```python
from build123d import *

# Parameters (mm, degrees)
F1_DEPTH = 50
F3_DEPTH = 3
F5_DEPTH = 3


with BuildPart() as f1:
    # F0 (on Front) → F1 (new body)
    with BuildSketch(Plane.XZ):
        Polygon((300, 0), (0, 0), (0, -3), (298.757359, -3), (474.655375, -178.898016), (476.776695, -176.776695), align=None)
    extrude(amount=F1_DEPTH)

    # F2 (on face) → F3 (join)
    with BuildSketch(Plane.XZ.offset(50)):
        Polygon((474.655375, -178.898016), (298.757359, -3), (0, -3), (0, -50), (279.289322, -50), (441.421356, -212.132034), align=None)
    extrude(amount=-F3_DEPTH)

    # F4 (on face) → F5 (join)
    with BuildSketch(Plane(origin=(0, 0, 0), x_dir=(-1, 0, 0), z_dir=(0, 1, 0))):
        Polygon((-298.757359, -3), (-474.655375, -178.898016), (-441.421356, -212.132034), (-279.289322, -50), (0, -50), (0, -3), align=None)
    extrude(amount=-F5_DEPTH)


solid = f1.part
```
Can you work these out from the model? Positions are in its coordinate system, mm. A direction names the side the tool comes from. Give positions to 0.01 mm unless a question says otherwise; leave off trailing zeros. Loops run counter-clockwise (first coordinate to the right, second up) from the corner with the lowest first, then second, coordinate; pieces in that order, holes last. Notation, with made-up numbers: M -4.5,67.5 L 53.5,67.5 A35 cw 53.5,101.5 Z; hole C 56.25,-10.5 d2. An arc over 180 degrees is marked long. Use one line per item in the form item = value. Start each with the question number.
(1) Please list where these lines run through material, in increasing order: line 1 (Y direction, x = 345, z = -78.5); line 2 (Z direction, x = 57.5, y = -46); line 3 (X direction, y = -44, z = -57.5).
(2) I'm going to push flat-ended pins straight in: P1, Ø2.5, axis at x = 172.5, y = -48, coming from the -Z side; P2, Ø4, axis at y = -31.5, z = -103.5, coming from the +X side; P3, Ø22, axis at x = 117, y = -33.5, coming from the -Z side. Where does each tip first touch, or does it pass through?
(3) I want a section at B-B, the plane y = -9. Write out the boundary of the cut face in (x, z), and give its area (3 significant figures).
(4) Thinking about a two-plate mould opening in Y: for faces 1 (the flat face through (237, -50, -43)), 2 (the flat face through (257, 0, -43)), 3 (the flat face through (385.48, -24.69, -89.72)), which applies, released by +Y, released by -Y, zero draft, split by the parting line, or undercut?
(5) On a 3-axis mill with a long thin cutter (end or side, diameter ignored), from which of +Z, -Z, +X, -X, +Y, -Y can I reach the whole of each face in a straight line? I mean faces 4 (the flat face through (256, -3, -45)), 5 (the flat face through (359.22, -48.52, -129.93)). Say none if no direction works.
(6) I want a section at C-C, the plane z = -33.5. Write out the boundary of the cut face in (x, y), and give its area (3 significant figures).
(7) I want a section at A-A, the plane x = 162. Write out the boundary of the cut face in (y, z), and give its area (3 significant figures).
Worked out:
q1.line_1 = -50 to -47, -3 to 0
q1.line_2 = -3 to 0
q1.line_3 = 353.26 to 357.5
q2.P1 = -50
q2.P2 = 405.5
q2.P3 = -3
q3.outline = M 0,-3 L 298.76,-3 L 474.66,-178.9 L 476.78,-176.78 L 300,0 L 0,0 Z
q3.area = 1,650 mm²
q4.face_1 = released by -Y
q4.face_2 = released by +Y
q4.face_3 = undercut
q5.face_4 = -Z, -X
q5.face_5 = -Z, -X, +Y, -Y
q6.outline = M 0,-50 L 333.5,-50 L 333.5,0 L 0,0 L 0,-3 L 329.26,-3 L 329.26,-47 L 0,-47 Z
q6.area = 2,190 mm²
q7.outline = M -50,-50 L -47,-50 L -47,-3 L -3,-3 L -3,-50 L 0,-50 L 0,0 L -50,0 Z
q7.area = 432 mm²
